from build123d import *

# Parameters (mm, degrees)
F0_W     = 28.08589302
F0_H     = 27.4060983211
F1_DEPTH = 3.81
F2_R     = 6.3416120596
F3_DEPTH = 7.62
F4_T     = -2.286


with BuildPart() as f1:
    # F0 (on Top) → F1 (new body)
    with BuildSketch(Plane.XY):
        Rectangle(F0_W, F0_H)
    extrude(amount=F1_DEPTH)

    # F2 (on Top) → F3 (join)
    with BuildSketch(Plane.XY):
        with Locations((-6.9529586472, 6.5272971988)):
            Circle(F2_R)
        with Locations((6.8254987709, 6.7306994461)):
            Circle(F2_R)
        with Locations((7.2046923451, -6.9202962331)):
            Circle(F2_R)
        with Locations((-7.015094161, -6.9202962331)):
            Circle(F2_R)
    extrude(amount=F3_DEPTH)

    # F4
    f4_openings = [f1.faces().sort_by_distance(p)[0] for p in [
        (-6.952959, 6.527297, 7.62),
        (-7.015094, -6.920296, 7.62),
        (7.204692, -6.920296, 7.62),
        (6.825499, 6.730699, 7.62),
    ]]
    offset(amount=F4_T, openings=f4_openings, kind=Kind.INTERSECTION)


solid = f1.part
Input: part model. Units: mm. Frame: model coordinates. A direction names the side the tool comes from. Round coordinates to 2 decimals unless told otherwise and drop trailing zeros. Loops run counter-clockwise (first coordinate to the right, second up) from the corner with the lowest first, then second, coordinate; pieces in that order, holes last. Notation, with made-up numbers: (43, -16.75) -> (62, -16.75) arc R20 ccw to (62, 1.25) -> close; hole circle Ø5 at (-0.75, 77). An arc over 180 degrees is marked (long way). Answer as a JSON object with one key per item and string values. Group by question number.
1) Section query A-A on z = 6.75. Output: boundary loops of the cut face in (x, y).
2) Section query D-D on z = 2.75. Output: boundary loops of the cut face in (x, y).
3) Section query B-B on x = -2. Output: boundary loops of the cut face in (y, z), plus the area to 3 significant figures.
4) Section query C-C on y = -7.25. Output: boundary loops of the cut face in (x, z).
5) Ray query, L1, parallel to X at y = -8, z = 4.25; L2, parallel to X at y = 4.5, z = 4.75; L3, parallel to X at y = 5.75, z = 3.5. Return the intervals inside material, ascending.
6) Pin query (flat end, axial travel): pin 1 (2.5 mm diameter, centred on x = -8, y = 7, fed in from +Z); pin 2 (4 mm diameter, centred on y = 3, z = 6, fed in from -X). Return the tip coordinate at first contact, or that it passes through.
7) Reachability of faces 4 (the cylindrical face through (-8.328, 0.336, 5.688)), 5 (the flat face through (0, 0, 0)) from +Z, -Z, +X, -X, +Y, -Y: full face, straight path, thin tool, end or side. Return the list, or none.
8) Draft query along Y for faces 1 (the flat face through (-7, 7, 2.286)), 2 (the flat face through (0, 13.703, 2)), 3 (the flat face through (-14.043, 0, 2)). Return one class per face: +Y half, -Y half, draft (parallel to the pull), parting line (faces both ways), or undercut.
Reply:
{
 "1": {"outline": "circle Ø12.68 at (-7.02, -6.92); circle Ø12.68 at (-6.95, 6.53); circle Ø12.68 at (6.83, 6.73); circle Ø12.68 at (7.2, -6.92); hole circle Ø8.11 at (-7.02, -6.92); hole circle Ø8.11 at (-6.95, 6.53); hole circle Ø8.11 at (6.83, 6.73); hole circle Ø8.11 at (7.2, -6.92)"},
 "2": {"outline": "(-14.04, -13.7) -> (14.04, -13.7) -> (14.04, 13.7) -> (-14.04, 13.7) -> close; hole circle Ø8.11 at (-7.02, -6.92); hole circle Ø8.11 at (-6.95, 6.53); hole circle Ø8.11 at (6.83, 6.73); hole circle Ø8.11 at (7.2, -6.92)"},
 "3": {"outline": "(-13.7, 0) -> (13.7, 0) -> (13.7, 3.81) -> (10.49, 3.81) -> (10.49, 7.62) -> (2.57, 7.62) -> (2.57, 3.81) -> (-3.04, 3.81) -> (-3.04, 7.62) -> (-10.8, 7.62) -> (-10.8, 3.81) -> (-13.7, 3.81) -> close", "area": "164 mm2"},
 "4": {"outline": "(-14.04, 0) -> (14.04, 0) -> (14.04, 3.81) -> (13.54, 3.81) -> (13.54, 7.62) -> (11.25, 7.62) -> (11.25, 2.29) -> (3.16, 2.29) -> (3.16, 7.62) -> (0.87, 7.62) -> (0.87, 3.81) -> (-0.68, 3.81) -> (-0.68, 7.62) -> (-2.97, 7.62) -> (-2.97, 2.29) -> (-11.06, 2.29) -> (-11.06, 7.62) -> (-13.35, 7.62) -> (-13.35, 3.81) -> (-14.04, 3.81) -> close"},
 "5": {"L1": "x = -13.26 to -10.92, -3.11 to -0.77, 0.96 to 3.3, 11.11 to 13.45", "L2": "x = -12.96 to -10.47, -3.44 to -0.94, 0.89 to 3.44, 10.21 to 12.76", "L3": "x = -14.04 to -10.93, -2.97 to 2.89, 10.76 to 14.04"},
 "6": {"pin 1": "stops at z = 2.29", "pin 2": "stops at x = -13.11"},
 "7": {"face 4": "+Z", "face 5": "-Z, +X, -X, +Y, -Y"},
 "8": {"face 1": "undercut", "face 2": "+Y half", "face 3": "draft"}
}
